Work out the finished part from the listing and answer in its coordinate system (mm). Face numbers are marked on the shaded views. Coordinates: 2 decimals unless noted, no trailing zeros. Order: outer loops, then holes, each group sorted by start corner. A loop starts at its lowest first (then second) coordinate and runs counter-clockwise, first axis right, second up. Notation, with made-up numbers: M 54.25,46 L 88.25,46 A15 ccw 88.25,52 Z; hole C 58.25,57 d1. An arc over 180 degrees is marked long. Answer in a Markdown table with one row per item. Add a question column.
Item 1: The part is cut by section C-C (z = 153.5). Write down the section's boundary in (x, y), then the cut area to 3 significant figures.
Item 2: The mould has two halves that part along X. Classify the marked faces 1, 2 and 3: released by +X, released by -X, zero draft, split by the parting line, or undercut.
Item 3: The part is cut by section A-A (y = 0). Write down the section's boundary in (x, z), then the cut area to 3 significant figures.
Item 4: Flat-ended cylindrical pins translate along their axes: pin 1 Ø1 at (x, y) = (-12.5, -15.5) entering from -Z; pin 2 Ø22 at (x, z) = (1, 165) entering from -Y; pin 3 Ø6 at (x, z) = (0, 43) entering from +Y; pin 4 Ø6 at (y, z) = (-8.5, 118) entering from +X. Find the tip coordinate at first contact, or state that the pin passes through.
Item 5: The part is cut by section B-B (x = 0). Write down the section's boundary in (y, z).
Item 6: Consider line 1 (Z direction, x = 21.5, y = 0); line 2 (Y direction, x = -3.5, z = 153); line 3 (X direction, y = -1, z = 126). Determine where each line is inside the solid, lowest interval first. Write a range as from..to.
Item 7: The part is cut by section D-D (z = 42). Write down the section's boundary in (x, y).
from build123d import *

# Parameters (mm, degrees)
IZIM2_R                     = 32.5
Y_KSEKLIK_EKSTR_ZYON1_DEPTH = 150
IZIM3_W                     = 20
IZIM3_H                     = 20
Y_KSEKLIK_EKSTR_ZYON2_DEPTH = 20
IZIM5_W                     = 20
IZIM5_H                     = 20
KES_EKSTR_ZYON2_DEPTH       = 20
IZIM6_W                     = 20.1
IZIM6_H                     = 20.1
KES_EKSTR_ZYON3_DEPTH       = 20


with BuildPart() as part:
    # Çizim2 → Yükseklik-Ekstrüzyon1 (new body)
    with BuildSketch(Plane.XY):
        Circle(IZIM2_R)
    extrude(amount=Y_KSEKLIK_EKSTR_ZYON1_DEPTH)

    # Çizim3 → Yükseklik-Ekstrüzyon2 (add)
    with BuildSketch(Plane.XY.offset(150)):
        Rectangle(IZIM3_W, IZIM3_H)
    extrude(amount=Y_KSEKLIK_EKSTR_ZYON2_DEPTH)

    # Çizim5 → Kes-Ekstrüzyon2 (cut)
    with BuildSketch(Plane(origin=(0, 0, 0), x_dir=(-1, 0, 0), z_dir=(0, 0, -1))):
        with Locations((0, 0.232689455)):
            Rectangle(IZIM5_W, IZIM5_H)
    extrude(amount=-KES_EKSTR_ZYON2_DEPTH, mode=Mode.SUBTRACT)

    # Çizim6 → Kes-Ekstrüzyon3 (cut)
    with BuildSketch(Plane(origin=(0, 0, 0), x_dir=(-1, 0, 0), z_dir=(0, 0, -1))):
        with Locations((0, 0.232689455)):
            Rectangle(IZIM6_W, IZIM6_H)
    extrude(amount=-KES_EKSTR_ZYON3_DEPTH, mode=Mode.SUBTRACT)


solid = part.part
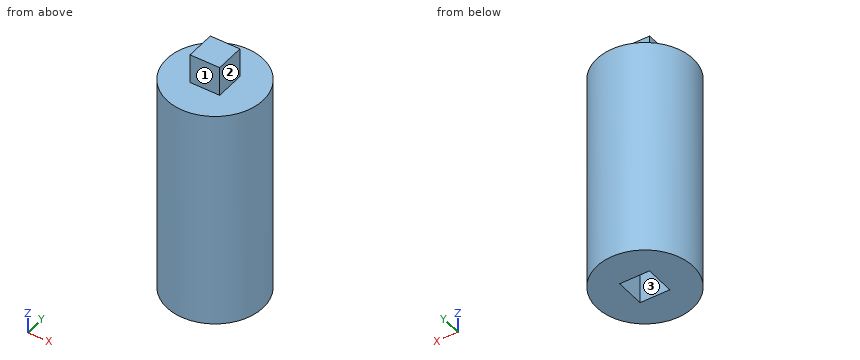
Reply:
| question | item | result |
|---|---|---|
| 1 | outline | M -10,-10 L 10,-10 L 10,10 L -10,10 Z |
| 1 | area | 400 mm2 |
| 2 | face 1 | zero draft |
| 2 | face 2 | released by +X |
| 2 | face 3 | undercut |
| 3 | outline | M -32.5,0 L -10.05,0 L -10.05,20 L 10.05,20 L 10.05,0 L 32.5,0 L 32.5,150 L 10,150 L 10,170 L -10,170 L -10,150 L -32.5,150 Z |
| 3 | area | 9,750 mm2 |
| 4 | pin 1 | stops at z = 0 |
| 4 | pin 2 | stops at y = -10 |
| 4 | pin 3 | stops at y = 32.5 |
| 4 | pin 4 | stops at x = 32.03 |
| 5 | outline | M -32.5,0 L -9.82,0 L -9.82,20 L 10.28,20 L 10.28,0 L 32.5,0 L 32.5,150 L 10,150 L 10,170 L -10,170 L -10,150 L -32.5,150 Z |
| 6 | line 1 | z = 0..150 |
| 6 | line 2 | y = -10..10 |
| 6 | line 3 | x = -32.48..32.48 |
| 7 | outline | C 0,0 d65 |
